Work out the finished part from the listing and answer in its coordinate system (mm). Face numbers are marked on the shaded views. A direction names the side the tool comes from. Give positions to 0.01 mm unless a question says otherwise; leave off trailing zeros. Loops run counter-clockwise (first coordinate to the right, second up) from the corner with the lowest first, then second, coordinate; pieces in that order, holes last. Notation, with made-up numbers: M -34.5,39.25 L -17.5,39.25 A25 ccw -17.5,61.25 Z; hole C 41.25,70 d2. An arc over 180 degrees is marked long. Use a Markdown table: item, result.
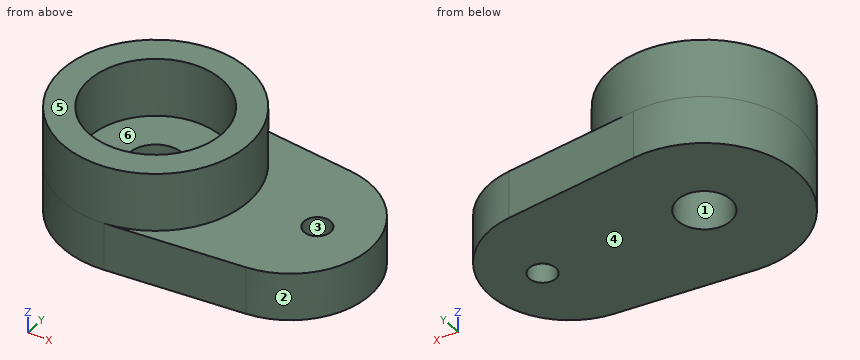
```python
from build123d import *

# Parameters (mm, degrees)
SKETCH1_R           = 1
SKETCH1_R_2         = 0.5
BOSS_EXTRUDE3_DEPTH = 1.8
SKETCH4_R           = 3.5
SKETCH4_R_2         = 2.5
BOSS_EXTRUDE4_DEPTH = 2.2


with BuildPart() as part:
    # Sketch1 → Boss-Extrude3 (new body)
    with BuildSketch(Plane.XY):
        with BuildLine():
            Line((0.35, 3.48245603), (5.3, 2.984962311))
            ThreePointArc((5.3, 2.984962311), (8, 0), (5.3, -2.984962311))
            Line((5.3, -2.984962311), (0.35, -3.48245603))
            ThreePointArc((0.35, -3.48245603), (-3.5, 0), (0.35, 3.48245603))
        make_face()
        Circle(SKETCH1_R, mode=Mode.SUBTRACT)
        with Locations((6, 0)):
            Circle(SKETCH1_R_2, mode=Mode.SUBTRACT)
    extrude(amount=BOSS_EXTRUDE3_DEPTH)

    # Sketch4 → Boss-Extrude4 (add)
    with BuildSketch(Plane.XY.offset(1.8)):
        with Locations(Location((0, 0, 0), (0, 0, 275.739170477))):
            Circle(SKETCH4_R)
        Circle(SKETCH4_R_2, mode=Mode.SUBTRACT)
    extrude(amount=BOSS_EXTRUDE4_DEPTH)


solid = part.part
```
(1) A cutting plane is placed at D-D (y = -1.75). Write down the section's boundary in (x, z).
Entries:
| item | result |
|---|---|
| outline | M -3.03,0 L 7.44,0 L 7.44,1.8 L 3.03,1.8 L 3.03,4 L 1.79,4 L 1.79,1.8 L -1.79,1.8 L -1.79,4 L -3.03,4 Z |
(2) A cutting plane is placed at C-C (z = 1.6). Write down the section's boundary in (x, y).
Entries:
| item | result |
|---|---|
| outline | M 0.35,-3.48 L 5.3,-2.98 A3 ccw 5.3,2.98 L 0.35,3.48 A3.5 ccw long Z; hole C 0,0 d2; hole C 6,0 d1 |
(3) Given P1, Ø3, axis at x = 0, y = 0, coming from the +Z side; P2, Ø1.5, axis at x = -1.5, z = 1, coming from the +Y side; P3, Ø1.8, axis at x = 0, y = 0, coming from the -Z side, each flat-ended and moving along its own axis, determine where each tip first touches the part or whether it passes through.
Entries:
| item | result |
|---|---|
| P1 | stops at z = 1.8 |
| P2 | stops at y = 3.42 |
| P3 | passes through |
(4) Which of the six approach directions +Z, -Z, +X, -X, +Y, -Y give full straight-line access (tool end or side, diameter ignored) to the marked faces 5 and 6?
Entries:
| item | result |
|---|---|
| face 5 | +Z, +X, -X, +Y, -Y |
| face 6 | +Z |
(5) Consider probe 1 along X at (y, z) = (0.25, 1.55); probe 2 along Z at (x, y) = (2.25, -1); probe 3 along X at (y, z) = (0.75, 0.35). Determine where each line is inside the solid, lowest interval first. Write a range as [from, to].
Entries:
| item | result |
|---|---|
| probe 1 | x = [-3.49, -0.97], [0.97, 5.57], [6.43, 7.99] |
| probe 2 | z = [0, 1.8] |
| probe 3 | x = [-3.42, -0.66], [0.66, 7.9] |
(6) The mould has two halves that part along X. Classify the marked faces 1, 2, 3 and 4: released by +X, released by -X, zero draft, split by the parting line, or undercut.
Entries:
| item | result |
|---|---|
| face 1 | undercut |
| face 2 | released by +X |
| face 3 | undercut |
| face 4 | zero draft |
(7) A cutting plane is placed at B-B (y = 0). Write down the section's boundary in (x, z), and give its area (3 significant figures).
Entries:
| item | result |
|---|---|
| outline | M -3.5,0 L -1,0 L -1,1.8 L -2.5,1.8 L -2.5,4 L -3.5,4 Z; M 1,0 L 5.5,0 L 5.5,1.8 L 3.5,1.8 L 3.5,4 L 2.5,4 L 2.5,1.8 L 1,1.8 Z; M 6.5,0 L 8,0 L 8,1.8 L 6.5,1.8 Z |
| area | 19.7 mm² |
(8) A cutting plane is placed at A-A (x = 0). Write down the section's boundary in (y, z), and give its area (3 significant figures).
Entries:
| item | result |
|---|---|
| outline | M -3.5,0 L -1,0 L -1,1.8 L -2.5,1.8 L -2.5,4 L -3.5,4 Z; M 1,0 L 3.5,0 L 3.5,4 L 2.5,4 L 2.5,1.8 L 1,1.8 Z |
| area | 13.4 mm² |
